Source: CAD feature listing. Evaluate the final solid. Frame: model axes, mm. A direction names the side the tool comes from. Coordinates: 2 decimals unless noted, no trailing zeros. Order: outer loops, then holes, each group sorted by start corner. A loop starts at its lowest first (then second) coordinate and runs counter-clockwise, first axis right, second up.
```python
from build123d import *

# Parameters (mm, degrees)
SKETCH1_W               = 13
SKETCH1_H               = 6
SKETCH1_R               = 1.5
BOSS_EXTRUDE1_DEPTH     = 4
BOSS_EXTRUDE1_2_DEPTH   = 4
BOSS_EXTRUDE2_START     = 4
SKETCH1_4_R             = 1.5
SKETCH1_4_W             = 13
SKETCH1_4_H             = 6
BOSS_EXTRUDE2_DEPTH     = 8
SKETCH2_R               = 1.5
BOSS_EXTRUDE3_DEPTH     = 5
SKETCH2_3_R             = 1.5
BOSS_EXTRUDE4_DEPTH     = 5
CUT_EXTRUDE1_DEPTH      = 3
FILLET3_R               = 3
SKETCH4_R               = 20.5
CUT_EXTRUDE2_DEPTH      = 6
CUT_EXTRUDE2_DEPTH_BACK = 13


with BuildPart() as part:
    # Sketch1 → Boss-Extrude1 (new body)
    with BuildSketch(Plane(origin=(0, -9, 0), x_dir=(1, 0, 0), z_dir=(0, 1, 0))):
        with Locations((25.1, 41)):
            Rectangle(SKETCH1_W, SKETCH1_H)
        with Locations((27.1, 41)):
            Circle(SKETCH1_R, mode=Mode.SUBTRACT)
        with Locations((23.1, 41)):
            Circle(SKETCH1_R, mode=Mode.SUBTRACT)
    extrude(amount=BOSS_EXTRUDE1_DEPTH)



with BuildPart() as body_2:
    # Sketch1 → Boss-Extrude1 2 (new body)
    with BuildSketch(Plane(origin=(0, -9, 0), x_dir=(1, 0, 0), z_dir=(0, 1, 0))):
        with BuildLine():
            ThreePointArc((22.6, 10.089722494), (23.395394249, 8.075767946), (24.01171589, 6))
            Line((24.01171589, 6), (35.6, 6))
            Line((35.6, 6), (35.6, 10.18070798))
            ThreePointArc((35.6, 10.18070798), (34.768444056, 11.068532406), (33.986085046, 12))
            Line((33.986085046, 12), (31.6, 12))
            Line((31.6, 12), (22.6, 12))
            Line((22.6, 12), (22.6, 10.089722494))
        make_face()
        with Locations((27.1, 9)):
            Circle(SKETCH1_R, mode=Mode.SUBTRACT)
        with Locations((31.1, 9)):
            Circle(SKETCH1_R, mode=Mode.SUBTRACT)
    extrude(amount=BOSS_EXTRUDE1_2_DEPTH)


with BuildPart() as part_1:
    add(part.part)

    add(body_2.part)  # Boss-Extrude2 merges body 2
    # Sketch1<4> → Boss-Extrude2 (add)
    with BuildSketch(Plane(origin=(0, -9, 0), x_dir=(1, 0, 0), z_dir=(0, 1, 0)).offset(BOSS_EXTRUDE2_START)):
        with BuildLine():
            ThreePointArc((22.6, 10.089722494), (23.395394249, 8.075767946), (24.01171589, 6))
            Line((24.01171589, 6), (35.6, 6))
            Line((35.6, 6), (35.6, 10.18070798))
            ThreePointArc((35.6, 10.18070798), (34.768444056, 11.068532406), (33.986085046, 12))
            Line((33.986085046, 12), (31.6, 12))
            Line((31.6, 12), (22.6, 12))
            Line((22.6, 12), (22.6, 10.089722494))
        make_face()
        with Locations((27.1, 9)):
            Circle(SKETCH1_4_R, mode=Mode.SUBTRACT)
        with Locations((31.1, 9)):
            Circle(SKETCH1_4_R, mode=Mode.SUBTRACT)
        with BuildLine():
            Line((21.646304534, 12), (22.6, 12))
            Line((22.6, 12), (31.6, 12))
            Line((31.6, 12), (31.6, 15.692235936))
            ThreePointArc((31.6, 15.692235936), (29.1, 26), (31.6, 36.307764064))
            Line((31.6, 36.307764064), (31.6, 38))
            Line((31.6, 38), (18.6, 38))
            Line((18.6, 38), (18.6, 16.327966805))
            ThreePointArc((18.6, 16.327966805), (20.239171953, 14.245645604), (21.646304534, 12))
        make_face()
        with BuildLine():
            Line((31.6, 15.692235936), (31.6, 12))
            Line((31.6, 12), (33.986085046, 12))
            ThreePointArc((33.986085046, 12), (32.702650951, 13.787702963), (31.6, 15.692235936))
        make_face()
        with BuildLine():
            ThreePointArc((21.646304534, 12), (22.143761114, 11.055150099), (22.6, 10.089722494))
            Line((22.6, 10.089722494), (22.6, 12))
            Line((22.6, 12), (21.646304534, 12))
        make_face()
        with Locations((25.1, 41)):
            Rectangle(SKETCH1_4_W, SKETCH1_4_H)
        with Locations((27.1, 41)):
            Circle(SKETCH1_4_R, mode=Mode.SUBTRACT)
        with Locations((23.1, 41)):
            Circle(SKETCH1_4_R, mode=Mode.SUBTRACT)
    extrude(amount=BOSS_EXTRUDE2_DEPTH)

    # Sketch2 → Boss-Extrude3 (add)
    with BuildSketch(Plane(origin=(0, 3, 0), x_dir=(1, 0, 0), z_dir=(0, 1, 0))):
        with BuildLine():
            ThreePointArc((32.6, 64), (37.6, 69), (42.6, 64))
            Line((42.6, 64), (42.6, 43))
            ThreePointArc((42.6, 43), (37.6, 38), (32.6, 43))
            Line((32.6, 43), (32.6, 64))
        make_face()
        with Locations((37.6, 64)):
            Circle(SKETCH2_R, mode=Mode.SUBTRACT)
        Polygon((24.675471698, 49.641509434), (30.1, 44), (31.6, 44), (32.6, 44), (32.6, 57), align=None)
        Polygon((24.675471698, 49.641509434), (18.6, 44), (30.1, 44), align=None)
        Polygon((30.1, 44), (18.6, 44), (18.6, 38), (31.6, 38), (31.6, 44), align=None)
        with Locations((23.1, 41)):
            Circle(SKETCH2_R, mode=Mode.SUBTRACT)
        with Locations((27.1, 41)):
            Circle(SKETCH2_R, mode=Mode.SUBTRACT)
        with BuildLine():
            Line((32.6, 43), (32.6, 38))
            Line((32.6, 38), (37.6, 38))
            ThreePointArc((37.6, 38), (34.064466094, 39.464466094), (32.6, 43))
        make_face()
        Polygon((32.6, 44), (31.6, 44), (31.6, 38), (32.6, 38), (32.6, 43), align=None)
    extrude(amount=BOSS_EXTRUDE3_DEPTH)

    # Sketch2<3> → Boss-Extrude4 (add)
    with BuildSketch(Plane(origin=(0, 3, 0), x_dir=(1, 0, 0), z_dir=(0, 1, 0))):
        with BuildLine():
            ThreePointArc((32.6, 64), (37.6, 69), (42.6, 64))
            Line((42.6, 64), (42.6, 43))
            ThreePointArc((42.6, 43), (37.6, 38), (32.6, 43))
            Line((32.6, 43), (32.6, 64))
        make_face()
        with Locations((37.6, 64)):
            Circle(SKETCH2_3_R, mode=Mode.SUBTRACT)
        Polygon((24.675471698, 49.641509434), (30.1, 44), (31.6, 44), (32.6, 44), (32.6, 57), align=None)
        Polygon((24.675471698, 49.641509434), (18.6, 44), (30.1, 44), align=None)
        Polygon((32.6, 44), (31.6, 44), (31.6, 38), (32.6, 38), (32.6, 43), align=None)
        with BuildLine():
            Line((32.6, 43), (32.6, 38))
            Line((32.6, 38), (37.6, 38))
            ThreePointArc((37.6, 38), (34.064466094, 39.464466094), (32.6, 43))
        make_face()
    extrude(amount=-BOSS_EXTRUDE4_DEPTH)

    # Sketch3 → Cut-Extrude1 (cut)
    with BuildSketch(Plane(origin=(0, 8, 0), x_dir=(1, 0, 0), z_dir=(0, 1, 0))):
        with BuildLine():
            Line((34.6, 60), (34.6, 56.127860975))
            Line((34.6, 56.127860975), (21.539226642, 44))
            Line((21.539226642, 44), (40.6, 44))
            Line((40.6, 44), (40.6, 60))
            ThreePointArc((40.6, 60), (37.6, 59), (34.6, 60))
        make_face()
    extrude(amount=-CUT_EXTRUDE1_DEPTH, mode=Mode.SUBTRACT)

    # Fillet3
    fillet3_edges = [part_1.edges().sort_by_distance(p)[0] for p in [
        (40.6, 6.5, -44),
        (21.539226642, 6.5, -44),
    ]]
    fillet(fillet3_edges, radius=FILLET3_R)

    # Sketch4 → Cut-Extrude2 (cut, two sides)
    with BuildSketch(Plane(origin=(0, 3, 0), x_dir=(1, 0, 0), z_dir=(0, 1, 0))) as cut_extrude2_sk:
        with Locations((51.6, 26)):
            Circle(SKETCH4_R)
    extrude(amount=CUT_EXTRUDE2_DEPTH, mode=Mode.SUBTRACT)
    extrude(cut_extrude2_sk.sketch, amount=-CUT_EXTRUDE2_DEPTH_BACK, mode=Mode.SUBTRACT)


solid = part_1.part
```
1. Section query A-A on y = 4. Return loops of the section in (x, z), plus the area to 3 significant figures.
Findings:
outline: (18.6, -44) - (32.6, -57) - (32.6, -64) arc R5 ccw to (42.6, -64) - (42.6, -44.42) arc R20.5 cw to (34.98, -38) - (18.6, -38) - close; hole circle Ø3 at (23.1, -41); hole circle Ø3 at (27.1, -41); hole circle Ø3 at (37.6, -64)
area: 425 mm2
2. Section query B-B on z = -9. Return loops of the section in (x, y), plus the area to 3 significant figures.
Findings:
outline: (23.06, -9) - (25.6, -9) - (25.6, 3) - (23.06, 3) - close; (28.6, -9) - (29.6, -9) - (29.6, 3) - (28.6, 3) - close; (32.6, -9) - (35.6, -9) - (35.6, 3) - (32.6, 3) - close
area: 78.5 mm2
3. Ray query, line 1 (Z direction, x = 27.1, y = -3.75); line 2 (Z direction, x = 31.1, y = -4); line 3 (X direction, y = -1.75, z = -41). Return the intervals inside material, ascending.
Findings:
line 1: z = -44 to -42.5, -39.5 to -10.5, -7.5 to -6
line 2: z = -44 to -35.27, -16.73 to -10.5, -7.5 to -6
line 3: x = 18.6 to 21.6, 24.6 to 25.6, 28.6 to 37.63
4. Draft query along X for faces 6 (the face through (24, -5, -27)), 7 (the face through (38.448, 2.93, -41.725)), 8 (the face through (33, 7, -44)). Return one class per face: released by +X, released by -X, zero draft, split by the parting line, or undercut.
Findings:
face 6: zero draft
face 7: released by +X
face 8: undercut
5. Section query C-C on y = 0.5. Return loops of the section in (x, z).
Findings:
outline: (18.6, -44) - (32.6, -57) - (32.6, -64) arc R5 ccw to (42.6, -64) - (42.6, -44.42) arc R20.5 cw to (34.98, -38) - (31.6, -38) - (31.6, -36.31) arc R22.5 cw to (35.6, -10.18) - (35.6, -6) - (24.01, -6) arc R24.75 cw to (18.6, -16.33) - close; hole circle Ø3 at (23.1, -41); hole circle Ø3 at (27.1, -41); hole circle Ø3 at (27.1, -9); hole circle Ø3 at (31.1, -9); hole circle Ø3 at (37.6, -64)
6. Section query D-D on x = 36.75. Return loops of the section in (y, z), plus the area to 3 significant figures.
Findings:
outline: (-2, -68.93) - (8, -68.93) - (8, -65.24) - (-2, -65.24) - close; (-2, -62.76) - (8, -62.76) - (8, -59.07) - (5, -59.07) - (5, -44) - (8, -44) - (8, -40.13) - (-2, -40.13) - close
area: 218 mm2
7. Pin query (flat end, axial travel): P1, Ø0.9, axis at y = 6, z = -50.5, coming from the -X side; P2, Ø1.8, axis at x = 31.1, z = -9, coming from the -Y side; P3, Ø7.5, axis at x = 25.5, y = -4.5, coming from the -Z side; P4, Ø8, axis at y = 0.5, z = -59.5, coming from the -X side. Return the tip coordinate at first contact, or that it passes through.
Findings:
P1: stops at x = 25.12
P2: passes through
P3: stops at z = -53
P4: stops at x = 30.98
8. Access query for faces 1 (the face through (35, 5, -50)), 2 (the face through (25, -7, -38)), 3 (the face through (32.6, 3, -60)), 4 (the face through (36.49, 2.93, -65.01)), 5 (the face through (42.6, 3, -54)). Directions: +Z, -Z, +X, -X, +Y, -Y. A direction counts if a zero-diameter tool reaches every point of the face in a straight line with its end or side. Return the directions, or none.
Findings:
face 1: +Y
face 2: +X, -X, -Y
face 3: -Z, -X, +Y, -Y
face 4: +Y, -Y
face 5: +Z, -Z, +X, +Y, -Y
